Answer from the drawing. Dimensions are ordinates in mm from the lowest x, y and z of the part. Round coordinates to 2 decimals unless told otherwise and drop trailing zeros. Write each loop counter-clockwise with the first axis right and the second up, starting at its lowest first coordinate (ties: lowest second). Pieces come first, ordered by that corner, then holes. Notation, with made-up numbers: (-14.75, -0.5) - (22.25, -0.5) arc R7 ccw to (22.25, 7.5) - close; hole circle Ø5 at (57, 21). An arc over 180 degrees is marked (long way). Return JSON: item names as keys, results as strings. Group by question number.
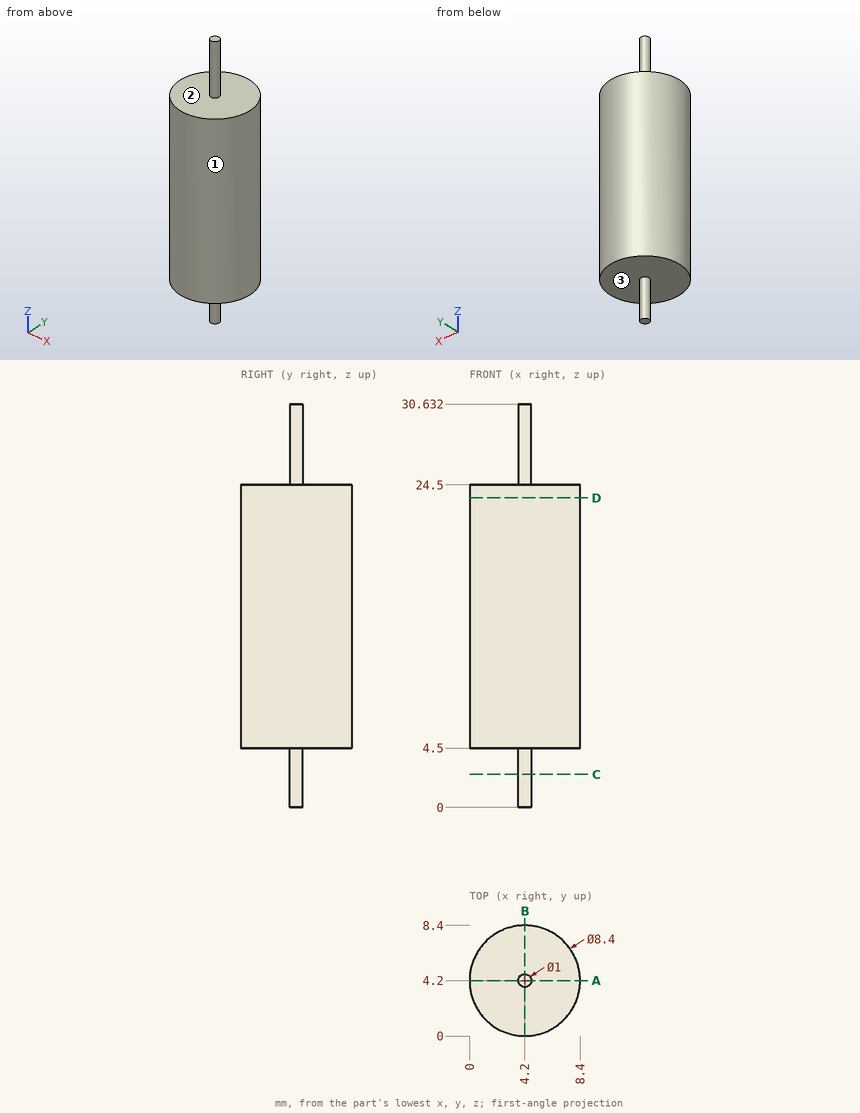
(1) Find section A-A (y = 4.2). Write down the section's boundary in (x, z).
(2) Find section C-C (z = 2.5). Write down the section's boundary in (x, y).
(3) Determine the mould class of the marked faces 1, 2 and 3 for opening direction Z: +Z half, -Z half, draft (parallel to the pull), parting line (faces both ways), or undercut.
(4) Consider line 1 (Z direction, x = 0.75, y = 3.5); line 2 (X direction, y = 4.25, z = 29.5). Determine where each line is inside the solid, lowest interval first.
(5) Find section D-D (z = 23.5). Write down the section's boundary in (x, y).
(6) Flat-ended cylindrical pins translate along their axes: pin 1 (5 mm diameter, centred on y = 7, z = 5.5, fed in from +X); pin 2 (1 mm diameter, centred on x = 6, z = 18, fed in from +Y); pin 3 (4 mm diameter, centred on x = 7.5, y = 1.5, fed in from -Z); pin 4 (1.5 mm diameter, centred on x = 2.5, z = 26, fed in from +Y). Find the tip coordinate at first contact, or state that the pin passes through.
Check sheet entries:
{
 "1": {"outline": "(0, 4.5) - (3.7, 4.5) - (3.7, 0) - (4.7, 0) - (4.7, 4.5) - (8.4, 4.5) - (8.4, 24.5) - (4.7, 24.5) - (4.7, 30.63) - (3.7, 30.63) - (3.7, 24.5) - (0, 24.5) - close"},
 "2": {"outline": "circle Ø1 at (4.2, 4.2)"},
 "3": {"face 1": "draft", "face 2": "+Z half", "face 3": "-Z half"},
 "4": {"line 1": "z = 4.5 to 24.5", "line 2": "x = 3.7 to 4.7"},
 "5": {"outline": "circle Ø8.4 at (4.2, 4.2)"},
 "6": {"pin 1": "stops at x = 8.39", "pin 2": "stops at y = 8.19", "pin 3": "stops at z = 4.5", "pin 4": "passes through"}
}
